```python
from build123d import *

# Parameters (mm, degrees)
F0_W     = 5.25
F0_H     = 5.25
F1_DEPTH = 5
F2_W     = 7
F2_H     = 7
F3_DEPTH = 1
F4_R     = 2
F5_DEPTH = 1.5


with BuildPart() as f1:
    # F0 (on Top) → F1 (new body)
    with BuildSketch(Plane.XY):
        Rectangle(F0_W, F0_H)
    extrude(amount=F1_DEPTH)

    # F2 (on face) → F3 (join)
    with BuildSketch(Plane.XY.offset(5)):
        Rectangle(F2_W, F2_H)
    extrude(amount=F3_DEPTH)

    # F4 (on face) → F5 (cut)
    with BuildSketch(Plane.XY.offset(6)):
        Circle(F4_R)
    extrude(amount=-F5_DEPTH, mode=Mode.SUBTRACT)


solid = f1.part
```
Geometry: final body of the model. Coordinates: model frame, mm. A direction names the side the tool comes from. Round coordinates to 2 decimals unless told otherwise and drop trailing zeros. Order: outer loops, then holes, each group sorted by start corner. A loop starts at its lowest first (then second) coordinate and runs counter-clockwise, first axis right, second up. Notation, with made-up numbers: (-17, 72.5) -> (-2, 72.5) arc R11 cw to (-2, 84.5) -> close; hole circle Ø11 at (70.5, -32.5). An arc over 180 degrees is marked (long way). Use CSV: the item, a comma, the result in double quotes. Start each with the question number.
1) Section B-B (x = -2.25). Return the cut outline in (y, z) (3 decimals).
2) Set-up query: faces 5 (the face through (2.625, 0, 2)), 6 (the face through (-2.625, 0, 2)), 7 (the face through (0, -2.625, 2)), 8 (the face through (0, 2.625, 2)). Return all of +Z, -Z, +X, -X, +Y, -Y with unobstructed straight access to the full face (end or side cutting, diameter ignored); none if empty.
3) Section A-A (z = 5.55). Return the cut outline in (x, y), and give its area (3 significant figures).
4) First-contact query: pin 1 Ø1.2 at (x, y) = (0, -0.5) entering from +Z; pin 2 Ø1.5 at (y, z) = (-1, 3.5) entering from -X (3 decimals). Flat tips, straight axial feed; report the tip coordinate or a pass-through.
5) Section C-C (y = -1). Return the cut outline in (x, z) (3 decimals), and give its area (3 significant figures).
6) Draft query along Y for faces 1 (the face through (0, -2, 5)), 2 (the face through (3.5, 0, 5.5)), 3 (the face through (0, 0, 4.5)), 4 (the face through (0, 3.5, 5.5)). Return one class per face: +Y half, -Y half, draft (parallel to the pull), parting line (faces both ways), or undercut.
7) Material intervals for line 1 along Y through (x, z) = (0, 5.2); line 2 along Y through (x, z) = (0, 4.9) (3 decimals); line 3 along Z through (x, y) = (2.75, -2), sorted ascending. Write a range as from..to.
8) Section D-D (z = 0.55). Return the cut outline in (x, y) (3 decimals), and give its area (3 significant figures).
Returned:
1,outline,"(-3.5, 5) -> (-2.625, 5) -> (-2.625, 0) -> (2.625, 0) -> (2.625, 5) -> (3.5, 5) -> (3.5, 6) -> (-3.5, 6) -> close"
2,face 5,"-Z, +X, +Y, -Y"
2,face 6,"-Z, -X, +Y, -Y"
2,face 7,"-Z, +X, -X, -Y"
2,face 8,"-Z, +X, -X, +Y"
3,outline,"(-3.5, -3.5) -> (3.5, -3.5) -> (3.5, 3.5) -> (-3.5, 3.5) -> close; hole circle Ø4 at (0, 0)"
3,area,"36.4 mm²"
4,pin 1,"stops at z = 4.5"
4,pin 2,"stops at x = -2.625"
5,outline,"(-3.5, 5) -> (-2.625, 5) -> (-2.625, 0) -> (2.625, 0) -> (2.625, 5) -> (3.5, 5) -> (3.5, 6) -> (1.732, 6) -> (1.732, 4.5) -> (-1.732, 4.5) -> (-1.732, 6) -> (-3.5, 6) -> close"
5,area,"28.1 mm²"
6,face 1,"undercut"
6,face 2,"draft"
6,face 3,"undercut"
6,face 4,"+Y half"
7,line 1,"y = -3.5..-2, 2..3.5"
7,line 2,"y = -2.625..-2, 2..2.625"
7,line 3,"z = 5..6"
8,outline,"(-2.625, -2.625) -> (2.625, -2.625) -> (2.625, 2.625) -> (-2.625, 2.625) -> close"
8,area,"27.6 mm²"
